from build123d import *

# Parameters (mm, degrees)
EXTRUDE_1_DEPTH       = 2
HOLE_WIZARD_M81_D     = 8.4
HOLE_WIZARD_M81_DEPTH = 2
CHAMFER_1_SIZE        = 2


with BuildPart() as part:
    # Эскиз1 → Бобышка-Вытянуть1 (new body)
    with BuildSketch(Plane(origin=(0, 0, 0), x_dir=(1, 0, 0), z_dir=(0, 0, -1))):
        Polygon((0, 0), (0, 160), (80, 160), (80, 80), (40, 0), align=None)
    extrude(amount=EXTRUDE_1_DEPTH)

    # Отверстие с зазором M81
    with Locations(Plane(origin=(0, 0, -2), x_dir=(1, 0, 0), z_dir=(0, 0, -1))):
        with Locations((20, 140), (20, 100), (20, 60), (20, 20), (60, 140), (60, 100)):
            Hole(HOLE_WIZARD_M81_D / 2, depth=HOLE_WIZARD_M81_DEPTH)

    # Фаска1
    chamfer_1_edges = [part.edges().sort_by_distance(p)[0] for p in [
        (0, 0, -1),
        (0, -160, -1),
        (80, -160, -1),
    ]]
    chamfer(chamfer_1_edges, length=CHAMFER_1_SIZE)


solid = part.part
Verification items for the finished model (mm, model axes). Coordinates: 2 decimals unless noted, no trailing zeros. Order: outer loops, then holes, each group sorted by start corner. A loop starts at its lowest first (then second) coordinate and runs counter-clockwise, first axis right, second up. Notation, with made-up numbers: M -0.75,-1 L 28.25,-1 A18 cw 28.25,4 Z; hole C 50.5,7.5 d4. An arc over 180 degrees is marked long. One line per item, written item: value. Start each with the question number.
Item 1: Mould release check, pull along X, two halves, no side actions. Record for faces 1 (the cylindrical face through (63.3, -97.4, -1)), 2 (the flat face through (41, -81, 0)), 3 (the flat face through (60.3, -40.6, -1)): pulls with the +X half, pulls with the -X half, needs draft (parallel to the pull), parting line crosses it, or undercut.
Item 2: Sectioned sample at D-D on z = -1.3. Record the cut outline in (x, y).
Item 3: Sectioned sample at B-B on x = 60. Record the cut outline in (y, z), then the cut area to 3 significant figures.
Item 4: Thickness scan on probe 1 along X at (y, z) = (-140, -1.05); probe 2 along Y at (x, z) = (20, -1.4); probe 3 along X at (y, z) = (-103, -0.5). Record the ranges inside material, lowest first.
Item 5: Sectioned sample at A-A on y = -60. Record the cut outline in (x, z), then the cut area to 3 significant figures.
Item 6: Sectioned sample at C-C on y = -100. Record the cut outline in (x, z).
Calculated:
1. face 1: undercut
1. face 2: needs draft
1. face 3: pulls with the +X half
2. outline: M 0,-158 L 2,-160 L 78,-160 L 80,-158 L 80,-80 L 40,0 L 2,0 L 0,-2 Z; hole C 20,-140 d8.4; hole C 20,-100 d8.4; hole C 20,-60 d8.4; hole C 20,-20 d8.4; hole C 60,-140 d8.4; hole C 60,-100 d8.4
3. outline: M -160,-2 L -144.2,-2 L -144.2,0 L -160,0 Z; M -135.8,-2 L -104.2,-2 L -104.2,0 L -135.8,0 Z; M -95.8,-2 L -40,-2 L -40,0 L -95.8,0 Z
3. area: 206 mm^2
4. probe 1: 0 to 15.8, 24.2 to 55.8, 64.2 to 80
4. probe 2: -160 to -144.2, -135.8 to -104.2, -95.8 to -64.2, -55.8 to -24.2, -15.8 to 0
4. probe 3: 0 to 17.06, 22.94 to 57.06, 62.94 to 80
5. outline: M 0,-2 L 15.8,-2 L 15.8,0 L 0,0 Z; M 24.2,-2 L 70,-2 L 70,0 L 24.2,0 Z
5. area: 123 mm^2
6. outline: M 0,-2 L 15.8,-2 L 15.8,0 L 0,0 Z; M 24.2,-2 L 55.8,-2 L 55.8,0 L 24.2,0 Z; M 64.2,-2 L 80,-2 L 80,0 L 64.2,0 Z
